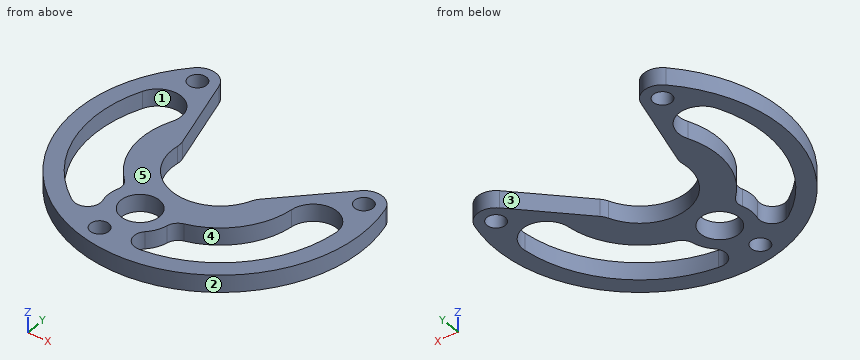
```python
from build123d import *

# Parameters (mm, degrees)
SKETCH1_R           = 2.15
BOSS_EXTRUDE1_DEPTH = 4
SKETCH2_R           = 4.5
CUT_EXTRUDE1_DEPTH  = 10
BOSS_EXTRUDE2_START = -4
SKETCH3_R           = 7.5
SKETCH3_R_2         = 4.5
BOSS_EXTRUDE2_DEPTH = 4
FILLET1_R           = 3


with BuildPart() as part:
    # Sketch1 → Boss-Extrude1 (new body)
    with BuildSketch(Plane.XY):
        with BuildLine():
            Line((169.071208826, 34.599951739), (155.49789847, 21.187541922))
            ThreePointArc((155.49789847, 21.187541922), (154.94043739, 20.512931345), (154.52928773, 19.740391219))
            ThreePointArc((154.52928773, 19.740391219), (141.205165824, 13.133334454), (132.969666153, 25.51727441))
            ThreePointArc((132.969666153, 25.51727441), (132.999870165, 26.391888614), (132.854399997, 27.254849052))
            Line((132.854399997, 27.254849052), (127.805773323, 45.656991858))
            ThreePointArc((127.805773323, 45.656991858), (124.72411503, 48.711211723), (120.534868929, 47.582011153))
            ThreePointArc((120.534868929, 47.582011153), (135.485264927, -8.213626307), (176.330506388, 32.631615154))
            ThreePointArc((176.330506388, 32.631615154), (173.267113127, 35.704154585), (169.071208826, 34.599951739))
        make_face()
        with Locations((123.610783427, 44.506096654)):
            Circle(SKETCH1_R, mode=Mode.SUBTRACT)
        with Locations((172.128729044, 31.505752308)):
            Circle(SKETCH1_R, mode=Mode.SUBTRACT)
        with Locations((136.611127773, -4.011848962)):
            Circle(SKETCH1_R, mode=Mode.SUBTRACT)
        with BuildLine():
            ThreePointArc((127.410923425, 31.346666741), (124.564673615, 38.661300157), (117.250040198, 35.815050347))
            ThreePointArc((117.250040198, 35.815050347), (115.76695708, 16.403661026), (126.757039397, 0.334446311))
            ThreePointArc((126.757039397, 0.334446311), (134.51482266, 1.526838378), (133.322430592, 9.284621641))
            ThreePointArc((133.322430592, 9.284621641), (126.488733751, 19.276552427), (127.410923425, 31.346666741))
        make_face(mode=Mode.SUBTRACT)
        with BuildLine():
            ThreePointArc((173.291771113, 20.798713806), (168.38023766, 26.920955155), (162.25799631, 22.009421702))
            ThreePointArc((162.25799631, 22.009421702), (157.021578838, 11.095301243), (146.107458379, 5.858883771))
            ThreePointArc((146.107458379, 5.858883771), (141.195924926, -0.263357578), (147.318166275, -5.174891032))
            ThreePointArc((147.318166275, -5.174891032), (164.870464109, 3.246415972), (173.291771113, 20.798713806))
        make_face(mode=Mode.SUBTRACT)
    extrude(amount=BOSS_EXTRUDE1_DEPTH)

    # Sketch2 → Cut-Extrude1 (cut)
    with BuildSketch(Plane(origin=(0, 0, 0), x_dir=(-1, 0, 0), z_dir=(0, 0, -1))):
        with Locations((-139.134613463, 5.405927844)):
            Circle(SKETCH2_R)
    extrude(amount=-CUT_EXTRUDE1_DEPTH, mode=Mode.SUBTRACT)

    # Sketch3 → Boss-Extrude2 (add)
    with BuildSketch(Plane.XY.offset(4).offset(BOSS_EXTRUDE2_START)):
        with Locations((139.134613463, 5.405927844)):
            Circle(SKETCH3_R)
        with Locations(Location((139.134613463, 5.405927844, 0), (0, 0, 180))):
            Circle(SKETCH3_R_2, mode=Mode.SUBTRACT)
    extrude(amount=BOSS_EXTRUDE2_DEPTH)

    # Fillet1
    fillet1_edges = [part.edges().sort_by_distance(p)[0] for p in [
        (133.49265497, 0.464439772, 2),
        (141.549948809, -1.694505605, 2),
        (146.616834445, 5.922037499, 2),
        (132.912874843, 9.594002408, 2),
    ]]
    fillet(fillet1_edges, radius=FILLET1_R)


solid = part.part
```
Geometry check sheet. Reference: the model listing, model coordinates, mm. Face numbers are marked on the shaded views. A direction names the side the tool comes from. Give positions to 0.01 mm unless a question says otherwise; leave off trailing zeros. Loops run counter-clockwise (first coordinate to the right, second up) from the corner with the lowest first, then second, coordinate; pieces in that order, holes last. Notation, with made-up numbers: M 2,55 L 26,55 A17 ccw 26,80 Z; hole C 56.5,86.25 d5. An arc over 180 degrees is marked long. Write item = value, one per line. Start each with the question number.
1. Go/stop test with flat-tipped pins: P1, Ø4, axis at x = 117.5, y = 24, coming from the +Z side; P2, Ø14.5, axis at x = 139.13, y = 5.41, coming from the +Z side. Record where each tip stops, or that it passes through.
2. Thickness scan on probe 1 along X at (y, z) = (3, 1.25); probe 2 along Y at (x, z) = (123.5, 2.7); probe 3 along X at (y, z) = (18, 3.6). Record the ranges inside material, lowest first.
3. Section check C-C, the plane x = 168. Enter the section's corners in (y, z).
4. Tool access check on the marked faces 4 and 5. Record the directions out of +Z, -Z, +X, -X, +Y, -Y that give a thin tool (end or side, any length) a straight path to the whole face; none if there is none.
5. Draft check along Y on the marked faces 1, 2 and 3. Enter one of: +Y half, -Y half, draft (parallel to the pull), parting line (faces both ways), or undercut.
6. Section check B-B, the plane y = 37. Enter the section's corners in (x, z).
7. Section check D-D, the plane z = 2.85. Give the number of separate pieces and of enclosed holes in the cut face, plus the area to 3 significant figures.
8. Section check A-A, the plane y = 24. Enter the section's corners in (x, z).
Values follow:
q1.P1 = through
q1.P2 = 4
q2.probe_1 = 118.21 to 123.61, 132.01 to 135.33, 142.94 to 146.24, 164.62 to 170.02
q2.probe_2 = -2.21 to 3.11, 39.01 to 42.36, 46.65 to 48.85
q2.probe_3 = 111.31 to 115.39, 126.88 to 134.6, 153.63 to 161.35, 172.85 to 176.92
q3.outline = M 0.72,0 L 6.94,0 L 6.94,4 L 0.72,4 Z; M 26.95,0 L 33.54,0 L 33.54,4 L 26.95,4 Z
q4.face_4 = +Z, -Z
q4.face_5 = +Z, +X, -X, +Y, -Y
q5.face_1 = undercut
q5.face_2 = parting line
q5.face_3 = +Y half
q6.outline = M 113.4,0 L 117.96,0 L 117.96,4 L 113.4,4 Z; M 126.7,0 L 130.18,0 L 130.18,4 L 126.7,4 Z
q7.separate_pieces = 1
q7.enclosed_holes = 6
q7.area = 1,130 mm^2
q8.outline = M 110.77,0 L 114.77,0 L 114.77,4 L 110.77,4 Z; M 125.87,0 L 132.87,0 L 132.87,4 L 125.87,4 Z; M 158.34,0 L 162.87,0 L 162.87,4 L 158.34,4 Z; M 172.68,0 L 177.47,0 L 177.47,4 L 172.68,4 Z
